The drawing under review shows one solid part. Ordinate dimensions are in mm from its lowest x, y, z. Give positions to 0.01 mm unless a question says otherwise; leave off trailing zeros. Loops run counter-clockwise (first coordinate to the right, second up) from the corner with the lowest first, then second, coordinate; pieces in that order, holes last. Notation, with made-up numbers: (48.5, -2.75) - (57.5, -2.75) arc R36 ccw to (57.5, 32.25) - close; hole circle Ø4 at (21, 20.25). An arc over 180 degrees is marked (long way). Write each question's results on one line, items separated by ' | '.
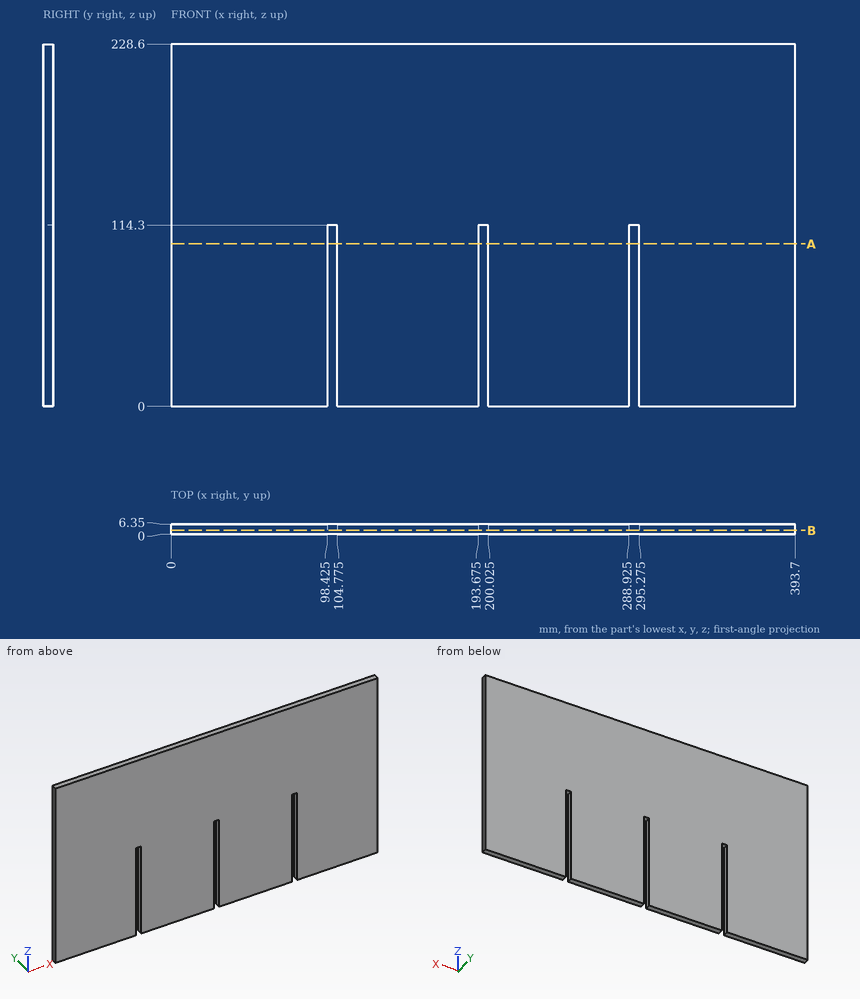
(1) Take a section at A-A on z = 102.5. Give the boundary of the cut face in (x, y) (3 decimals), plus the area to 3 significant figures.
Answers below:
outline: (0, 0) - (98.425, 0) - (98.425, 6.35) - (0, 6.35) - close; (104.775, 0) - (193.675, 0) - (193.675, 6.35) - (104.775, 6.35) - close; (200.025, 0) - (288.925, 0) - (288.925, 6.35) - (200.025, 6.35) - close; (295.275, 0) - (393.7, 0) - (393.7, 6.35) - (295.275, 6.35) - close | area: 2,380 mm2
(2) Wall thickness on line 1 along X through (y, z) = (5.25, 47.5) (3 decimals); line 2 along Z through (x, y) = (291, 4): over which ranges is each line inside the solid? List them lowest first. Write a range as from..to.
Answers below:
line 1: 0..98.425, 104.775..193.675, 200.025..288.925, 295.275..393.7 | line 2: 114.3..228.6
(3) Take a section at B-B on y = 2.5. Give the boundary of the cut face in (x, z) (3 decimals).
Answers below:
outline: (0, 0) - (98.425, 0) - (98.425, 114.3) - (104.775, 114.3) - (104.775, 0) - (193.675, 0) - (193.675, 114.3) - (200.025, 114.3) - (200.025, 0) - (288.925, 0) - (288.925, 114.3) - (295.275, 114.3) - (295.275, 0) - (393.7, 0) - (393.7, 228.6) - (0, 228.6) - close
(4) Insertion check: P1, Ø1.9, axis at x = 291, y = 3, coming from the -Z side. The pin has a flat end and moves straight along its axis. Give the tip position at first contact, or say it passes through.
Answers below:
P1: z = 114.3
